Geometry: final body of the model. Coordinates: model frame, mm. Face numbers are marked on the shaded views. Give positions to 0.01 mm unless a question says otherwise; leave off trailing zeros. Write each loop counter-clockwise with the first axis right and the second up, starting at its lowest first coordinate (ties: lowest second). Pieces come first, ordered by that corner, then holes. Notation, with made-up numbers: M 67.5,38 L 76.5,38 A30 cw 76.5,76 Z; hole C 18,84.5 d10. An arc over 180 degrees is marked long. Use a Markdown table: item, result. Add a question column.
(1) Cut plane A-A (z = -29). Output: boundary loops of the cut face in (x, y) (1 decimal), plus the area to 3 significant figures.
(2) Material intervals for L1, parallel to Y at x = -42, z = -17; L2, parallel to Y at x = 7, z = -27.5; L3, parallel to Z at x = -42, y = 1, sorted ascending.
(3) Draft query along X for the marked faces 1, 2 and 3. Return one class per face: released by +X, released by -X, zero draft, split by the parting line, or undercut.
(4) Cut plane B-B (z = -5.5). Output: boundary loops of the cut face in (x, y), plus the area to 3 significant figures.
(5) Pin query (flat end, axial travel): pin 1 Ø2 at (x, y) = (5, -9.5) entering from +Z; pin 2 Ø8 at (x, y) = (8, -9) entering from -Z; pin 3 Ø3 at (y, z) = (-10, -48) entering from +X; pin 4 Ø4 at (x, y) = (-28.5, -4) entering from +Z. Return the tip coordinate at first contact, or that it passes through.
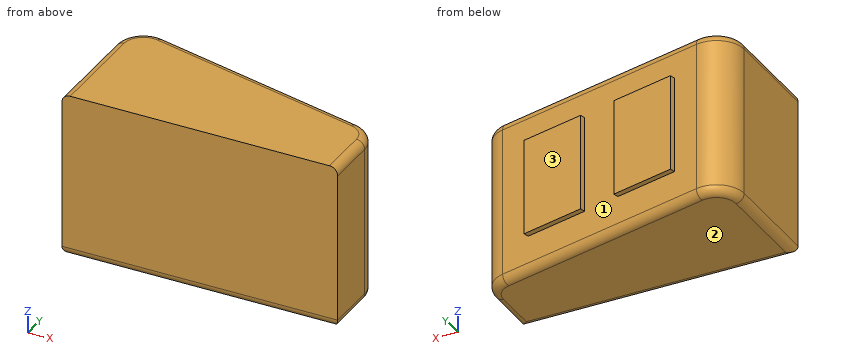
```python
from build123d import *

# Parameters (mm, degrees)
BOSS_EXTRUDE1_DEPTH = 60
SKETCH2_W           = 24
SKETCH2_H           = 35
BOSS_EXTRUDE2_DEPTH = 2
FILLET1_R           = 3


with BuildPart() as part:
    # Sketch1 → Boss-Extrude1 (new body)
    with BuildSketch(Plane.XY):
        with BuildLine():
            Line((-54.744118035, 4.205632013), (25.255881965, -14.454907336))
            ThreePointArc((25.255881965, -14.454907336), (30.817424359, -17.97721097), (32.984293194, -24.193484463))
            Line((32.984293194, -24.193484463), (32.984293194, -42.931937173))
            Line((32.984293194, -42.931937173), (-67.015706806, -42.931937173))
            Line((-67.015706806, -42.931937173), (-67.015706806, -5.532945114))
            ThreePointArc((-67.015706806, -5.532945114), (-63.2319803, 2.300186052), (-54.744118035, 4.205632013))
        make_face()
    extrude(amount=-BOSS_EXTRUDE1_DEPTH)

    # Sketch2 → Boss-Extrude2 (add)
    with BuildSketch(Plane(origin=(-1.894488045, -8.121900487, 0), x_dir=(0.9738577126840912, -0.22715887710083071, 0), z_dir=(0.22715887710083071, 0.9738577126840912, 0))):
        with Locations((-32.992105981, 29.5)):
            Rectangle(SKETCH2_W, SKETCH2_H)
        with Locations((5.084176419, 29.5)):
            Rectangle(SKETCH2_W, SKETCH2_H)
    extrude(amount=BOSS_EXTRUDE2_DEPTH)

    # Fillet1
    fillet1_edges = [part.edges().sort_by_distance(p)[0] for p in [
        (-14.744118035, -5.124637662, -60),
        (-63.2319803, 2.300186052, -60),
        (-67.015706806, -24.232441143, -60),
        (-17.015706806, -42.931937173, -60),
        (32.984293194, -33.562710818, -60),
        (-67.015706806, -24.232441143, 0),
        (-63.2319803, 2.300186052, 0),
        (-14.744118035, -5.124637662, 0),
        (30.817424359, -17.97721097, 0),
        (32.984293194, -33.562710818, 0),
        (30.817424359, -17.97721097, -60),
    ]]
    fillet(fillet1_edges, radius=FILLET1_R)


solid = part.part
```
Answer list:
| question | item | result |
|---|---|---|
| 1 | outline | M -67,-42.9 L 33,-42.9 L 33,-24.2 A10 ccw 25.3,-14.5 L 14.7,-12 L 15.2,-10.1 L -8.2,-4.6 L -8.6,-6.6 L -22.3,-3.4 L -21.9,-1.4 L -45.3,4 L -45.7,2.1 L -54.7,4.2 A10 ccw -67,-5.5 Z |
| 1 | area | 3,880 mm² |
| 2 | L1 | -42.93 to 3.29 |
| 2 | L2 | -42.93 to -8.14 |
| 2 | L3 | -58.14 to -1.86 |
| 3 | face 1 | undercut |
| 3 | face 2 | zero draft |
| 3 | face 3 | released by +X |
| 4 | outline | M -67.02,-42.93 L 32.98,-42.93 L 32.98,-24.19 A10 ccw 25.26,-14.45 L -54.74,4.21 A10 ccw -67.02,-5.53 Z |
| 4 | area | 3,790 mm² |
| 5 | pin 1 | z = -0.99 |
| 5 | pin 2 | z = -59.97 |
| 5 | pin 3 | x = 15.2 |
| 5 | pin 4 | z = 0 |
